```python
from build123d import *

# Parameters (mm, degrees)
BASE_FLANGE1_DEPTH             = 17.5
EDGE_FLANGE1_STRIP_W           = 4.4196
EDGE_FLANGE1_STRIP_H           = 0.7366
EDGE_FLANGE1_STRIP_CUT_DEPTH   = 445.0536
EDGE_FLANGE1_DEPTH             = 445.0536
EDGE_FLANGE2_STRIP_W           = 4.4196
EDGE_FLANGE2_STRIP_H           = 0.7366
EDGE_FLANGE2_STRIP_CUT_DEPTH   = 445.0536
EDGE_FLANGE2_DEPTH             = 445.0536
CUT_EXTRUDE1_DEPTH             = 512.790467768
CUT_EXTRUDE1_DEPTH_BACK        = 512.790467768
SKETCH16_R                     = 2
EDGE_FLANGE3_STRIP_W           = 4.4196
EDGE_FLANGE3_STRIP_H           = 0.7366
EDGE_FLANGE3_STRIP_CUT_DEPTH   = 97.7902
EDGE_FLANGE3_STRIP_2_W         = 4.4196
EDGE_FLANGE3_STRIP_2_H         = 0.7366
EDGE_FLANGE3_STRIP_CUT_2_DEPTH = 97.7902
EDGE_FLANGE3_DEPTH             = 97.7902
EDGE_FLANGE3_BEND_DEPTH        = 97.7902
EDGE_FLANGE4_STRIP_W           = 4.4196
EDGE_FLANGE4_STRIP_H           = 0.7366
EDGE_FLANGE4_STRIP_CUT_DEPTH   = 97.7902
EDGE_FLANGE4_STRIP_2_W         = 4.4196
EDGE_FLANGE4_STRIP_2_H         = 0.7366
EDGE_FLANGE4_STRIP_CUT_2_DEPTH = 97.7902
EDGE_FLANGE4_DEPTH             = 97.7902
EDGE_FLANGE4_BEND_DEPTH        = 97.7902
FILLET1_R                      = 5
FILLET2_R                      = 3
CUT_EXTRUDE2_DEPTH             = 271.508951016
CUT_EXTRUDE2_DEPTH_BACK        = 271.508951016
SKETCH29_R                     = 2.5
CUT_EXTRUDE3_DEPTH             = 271.508951016
CUT_EXTRUDE3_DEPTH_BACK        = 271.508951016
SKETCH30_R                     = 1


# Sheet-metal steps are written as plain solids
with BuildPart() as part:
    # Sketch1 → Base-Flange1 (new, symmetric)
    with BuildSketch(Plane.XY):
        with BuildLine():
            Line((-250, 74), (-250, 99.2634))
            ThreePointArc((-250, 99.2634), (-249.784254855, 99.784254855), (-249.2634, 100))
            Line((-249.2634, 100), (-224.7366, 100))
            ThreePointArc((-224.7366, 100), (-224.215745145, 99.784254855), (-224, 99.2634))
            Line((-224, 99.2634), (-224, 1.4732))
            ThreePointArc((-224, 1.4732), (-223.56850971, 0.43149029), (-222.5268, 0))
            Line((-222.5268, 0), (222.5268, 0))
            ThreePointArc((222.5268, 0), (223.56850971, 0.43149029), (224, 1.4732))
            Line((224, 1.4732), (224, 99.2634))
            ThreePointArc((224, 99.2634), (224.215745145, 99.784254855), (224.7366, 100))
            Line((224.7366, 100), (249.2634, 100))
            ThreePointArc((249.2634, 100), (249.784254855, 99.784254855), (250, 99.2634))
            Line((250, 99.2634), (250, 74))
            Line((250, 74), (250.7366, 74))
            Line((250.7366, 74), (250.7366, 99.2634))
            ThreePointArc((250.7366, 99.2634), (250.30510971, 100.30510971), (249.2634, 100.7366))
            Line((249.2634, 100.7366), (224.7366, 100.7366))
            ThreePointArc((224.7366, 100.7366), (223.69489029, 100.30510971), (223.2634, 99.2634))
            Line((223.2634, 99.2634), (223.2634, 1.4732))
            ThreePointArc((223.2634, 1.4732), (223.047654855, 0.952345145), (222.5268, 0.7366))
            Line((222.5268, 0.7366), (-222.5268, 0.7366))
            ThreePointArc((-222.5268, 0.7366), (-223.047654855, 0.952345145), (-223.2634, 1.4732))
            Line((-223.2634, 1.4732), (-223.2634, 99.2634))
            ThreePointArc((-223.2634, 99.2634), (-223.69489029, 100.30510971), (-224.7366, 100.7366))
            Line((-224.7366, 100.7366), (-249.2634, 100.7366))
            ThreePointArc((-249.2634, 100.7366), (-250.30510971, 100.30510971), (-250.7366, 99.2634))
            Line((-250.7366, 99.2634), (-250.7366, 74))
            Line((-250.7366, 74), (-250, 74))
        make_face()
    extrude(amount=BASE_FLANGE1_DEPTH, both=True)

    # Edge-Flange1 strip (across the edge) → Edge-Flange1 strip cut (cut)
    with BuildSketch(Plane(origin=(222.5268, 0, 17.5), x_dir=(0, 0, -1), z_dir=(-1, 0, 0))):
        with Locations((-0.7366, -0.3683)):
            Rectangle(EDGE_FLANGE1_STRIP_W, EDGE_FLANGE1_STRIP_H)
    extrude(amount=EDGE_FLANGE1_STRIP_CUT_DEPTH, mode=Mode.SUBTRACT)

    # Edge-Flange1 section (across the edge) → Edge-Flange1 (add)
    with BuildSketch(Plane(origin=(222.5268, 0, 17.5), x_dir=(0, 0, -1), z_dir=(-1, 0, 0))):
        with BuildLine():
            Line((0, 0.7366), (0, 9.2634))
            Line((0, 9.2634), (0.7366, 9.2634))
            Line((0.7366, 9.2634), (0.7366, 0.7366))
            ThreePointArc((0.7366, 0.7366), (0.952345145, 0.215745145), (1.4732, 0))
            Line((1.4732, 0), (1.4732, -0.7366))
            ThreePointArc((1.4732, -0.7366), (0.43149029, -0.30510971), (0, 0.7366))
        make_face()
    extrude(amount=EDGE_FLANGE1_DEPTH)

    # Edge-Flange2 strip (across the edge) → Edge-Flange2 strip cut (cut)
    with BuildSketch(Plane(origin=(-222.5268, 0, -17.5), x_dir=(0, 0, 1), z_dir=(1, 0, 0))):
        with Locations((-0.7366, -0.3683)):
            Rectangle(EDGE_FLANGE2_STRIP_W, EDGE_FLANGE2_STRIP_H)
    extrude(amount=EDGE_FLANGE2_STRIP_CUT_DEPTH, mode=Mode.SUBTRACT)

    # Edge-Flange2 section (across the edge) → Edge-Flange2 (add)
    with BuildSketch(Plane(origin=(-222.5268, 0, -17.5), x_dir=(0, 0, 1), z_dir=(1, 0, 0))):
        with BuildLine():
            Line((0, 0.7366), (0, 9.2634))
            Line((0, 9.2634), (0.7366, 9.2634))
            Line((0.7366, 9.2634), (0.7366, 0.7366))
            ThreePointArc((0.7366, 0.7366), (0.952345145, 0.215745145), (1.4732, 0))
            Line((1.4732, 0), (1.4732, -0.7366))
            ThreePointArc((1.4732, -0.7366), (0.43149029, -0.30510971), (0, 0.7366))
        make_face()
    extrude(amount=EDGE_FLANGE2_DEPTH)

    # Sketch16 → Cut-Extrude1 (cut, two sides: drawn at the far end of the back side and taken through both)
    with BuildSketch(Plane(origin=(250.7366, 0, 0), x_dir=(0, 0, -1), z_dir=(1, 0, 0)).offset(-CUT_EXTRUDE1_DEPTH_BACK)):
        with Locations(Location((0, 88.7366, 0), (0, 0, 180))):
            Circle(SKETCH16_R)
    extrude(amount=CUT_EXTRUDE1_DEPTH + CUT_EXTRUDE1_DEPTH_BACK, mode=Mode.SUBTRACT)

    # Edge-Flange3 strip (across the edge) → Edge-Flange3 strip cut (cut)
    with BuildSketch(Plane(origin=(-223.2634, 99.2634, 17.5), x_dir=(0, 0, -1), z_dir=(0, -1, 0))):
        with Locations((-0.7366, -0.3683)):
            Rectangle(EDGE_FLANGE3_STRIP_W, EDGE_FLANGE3_STRIP_H)
    extrude(amount=EDGE_FLANGE3_STRIP_CUT_DEPTH, mode=Mode.SUBTRACT)

    # Edge-Flange3 strip 2 (across the edge) → Edge-Flange3 strip cut 2 (cut)
    with BuildSketch(Plane(origin=(-223.2634, 1.4732, -17.5), x_dir=(0, 0, 1), z_dir=(0, 1, 0))):
        with Locations((-0.7366, -0.3683)):
            Rectangle(EDGE_FLANGE3_STRIP_2_W, EDGE_FLANGE3_STRIP_2_H)
    extrude(amount=EDGE_FLANGE3_STRIP_CUT_2_DEPTH, mode=Mode.SUBTRACT)

    # Edge-Flange3 section (across the edge) → Edge-Flange3 (add)
    with BuildSketch(Plane(origin=(-223.2634, 99.2634, 17.5), x_dir=(0, 0, -1), z_dir=(0, -1, 0))):
        with BuildLine():
            Line((0, 0.7366), (0, 9.2634))
            Line((0, 9.2634), (0.7366, 9.2634))
            Line((0.7366, 9.2634), (0.7366, 0.7366))
            ThreePointArc((0.7366, 0.7366), (0.952345145, 0.215745145), (1.4732, 0))
            Line((1.4732, 0), (1.4732, -0.7366))
            ThreePointArc((1.4732, -0.7366), (0.43149029, -0.30510971), (0, 0.7366))
        make_face()
    extrude(amount=EDGE_FLANGE3_DEPTH)

    # Edge-Flange3 section 2 (across the edge) → Edge-Flange3 bend (add)
    with BuildSketch(Plane(origin=(-223.2634, 1.4732, -17.5), x_dir=(0, 0, 1), z_dir=(0, 1, 0))):
        with BuildLine():
            Line((0, 0.7366), (0, 9.2634))
            Line((0, 9.2634), (0.7366, 9.2634))
            Line((0.7366, 9.2634), (0.7366, 0.7366))
            ThreePointArc((0.7366, 0.7366), (0.952345145, 0.215745145), (1.4732, 0))
            Line((1.4732, 0), (1.4732, -0.7366))
            ThreePointArc((1.4732, -0.7366), (0.43149029, -0.30510971), (0, 0.7366))
        make_face()
    extrude(amount=EDGE_FLANGE3_BEND_DEPTH)

    # Edge-Flange4 strip (across the edge) → Edge-Flange4 strip cut (cut)
    with BuildSketch(Plane(origin=(223.2634, 1.4732, 17.5), x_dir=(0, 0, -1), z_dir=(0, 1, 0))):
        with Locations((-0.7366, -0.3683)):
            Rectangle(EDGE_FLANGE4_STRIP_W, EDGE_FLANGE4_STRIP_H)
    extrude(amount=EDGE_FLANGE4_STRIP_CUT_DEPTH, mode=Mode.SUBTRACT)

    # Edge-Flange4 strip 2 (across the edge) → Edge-Flange4 strip cut 2 (cut)
    with BuildSketch(Plane(origin=(223.2634, 99.2634, -17.5), x_dir=(0, 0, 1), z_dir=(0, -1, 0))):
        with Locations((-0.7366, -0.3683)):
            Rectangle(EDGE_FLANGE4_STRIP_2_W, EDGE_FLANGE4_STRIP_2_H)
    extrude(amount=EDGE_FLANGE4_STRIP_CUT_2_DEPTH, mode=Mode.SUBTRACT)

    # Edge-Flange4 section (across the edge) → Edge-Flange4 (add)
    with BuildSketch(Plane(origin=(223.2634, 1.4732, 17.5), x_dir=(0, 0, -1), z_dir=(0, 1, 0))):
        with BuildLine():
            Line((0, 0.7366), (0, 9.2634))
            Line((0, 9.2634), (0.7366, 9.2634))
            Line((0.7366, 9.2634), (0.7366, 0.7366))
            ThreePointArc((0.7366, 0.7366), (0.952345145, 0.215745145), (1.4732, 0))
            Line((1.4732, 0), (1.4732, -0.7366))
            ThreePointArc((1.4732, -0.7366), (0.43149029, -0.30510971), (0, 0.7366))
        make_face()
    extrude(amount=EDGE_FLANGE4_DEPTH)

    # Edge-Flange4 section 2 (across the edge) → Edge-Flange4 bend (add)
    with BuildSketch(Plane(origin=(223.2634, 99.2634, -17.5), x_dir=(0, 0, 1), z_dir=(0, -1, 0))):
        with BuildLine():
            Line((0, 0.7366), (0, 9.2634))
            Line((0, 9.2634), (0.7366, 9.2634))
            Line((0.7366, 9.2634), (0.7366, 0.7366))
            ThreePointArc((0.7366, 0.7366), (0.952345145, 0.215745145), (1.4732, 0))
            Line((1.4732, 0), (1.4732, -0.7366))
            ThreePointArc((1.4732, -0.7366), (0.43149029, -0.30510971), (0, 0.7366))
        make_face()
    extrude(amount=EDGE_FLANGE4_BEND_DEPTH)

    # Fillet1
    fillet1_edges = [part.edges().sort_by_distance(p)[0] for p in [
        (222.5268, -9.2634, 17.1317),
        (-222.5268, -9.2634, 17.1317),
        (-222.5268, -9.2634, -17.1317),
        (222.5268, -9.2634, -17.1317),
        (-214, 99.2634, 17.1317),
        (250.3683, 74, -17.5),
        (-214, 99.2634, -17.1317),
        (-250.3683, 74, -17.5),
        (214, 99.2634, 17.1317),
        (214, 99.2634, -17.1317),
        (250.3683, 74, 17.5),
        (-250.3683, 74, 17.5),
    ]]
    fillet(fillet1_edges, radius=FILLET1_R)

    # Fillet2
    fillet2_edges = [part.edges().sort_by_distance(p)[0] for p in [
        (-214, 1.4732, 17.1317),
        (-214, 1.4732, -17.1317),
        (214, 1.4732, 17.1317),
        (214, 1.4732, -17.1317),
    ]]
    fillet(fillet2_edges, radius=FILLET2_R)

    # Sketch29 → Cut-Extrude2 (cut, two sides: drawn at the far end of the back side and taken through both)
    with BuildSketch(Plane(origin=(0, 0.7366, 0), x_dir=(1, 0, 0), z_dir=(0, 1, 0)).offset(-CUT_EXTRUDE2_DEPTH_BACK)):
        with Locations(Location((-26.25, 0, 0), (0, 0, 90))):
            Circle(SKETCH29_R)
        with Locations(Location((26.25, 0, 0), (0, 0, 90))):
            Circle(SKETCH29_R)
    extrude(amount=CUT_EXTRUDE2_DEPTH + CUT_EXTRUDE2_DEPTH_BACK, mode=Mode.SUBTRACT)

    # Sketch30 → Cut-Extrude3 (cut, two sides: drawn at the far end of the back side and taken through both)
    with BuildSketch(Plane(origin=(0, 0.7366, 0), x_dir=(1, 0, 0), z_dir=(0, 1, 0)).offset(-CUT_EXTRUDE3_DEPTH_BACK)):
        with Locations(Location((-14.1, 14.1, 0), (0, 0, 90))):
            Circle(SKETCH30_R)
        with Locations(Location((14.1, 14.1, 0), (0, 0, 90))):
            Circle(SKETCH30_R)
        with Locations(Location((14.1, -14.1, 0), (0, 0, 90))):
            Circle(SKETCH30_R)
        with Locations(Location((-14.1, -14.1, 0), (0, 0, 90))):
            Circle(SKETCH30_R)
    extrude(amount=CUT_EXTRUDE3_DEPTH + CUT_EXTRUDE3_DEPTH_BACK, mode=Mode.SUBTRACT)


solid = part.part
```
Work out the finished part from the listing and answer in its coordinate system (mm). A direction names the side the tool comes from. Give positions to 0.01 mm unless a question says otherwise; leave off trailing zeros. Loops run counter-clockwise (first coordinate to the right, second up) from the corner with the lowest first, then second, coordinate; pieces in that order, holes last. Notation, with made-up numbers: (46.25, 60.5) -> (100.25, 60.5) arc R21 ccw to (100.25, 89.5) -> close; hole circle Ø9 at (11, 66.25). An arc over 180 degrees is marked (long way). Put each result on its own line as item: value. Start each with the question number.
Item 1: The mould has two halves that part along Z. Classify faces 4 (the face through (-218, 51, 16.763)), 5 (the face through (218, 51, -17.5)), 6 (the face through (-224, 51, 0)): released by +Z, released by -Z, zero draft, split by the parting line, or undercut.
Item 2: Which of the six approach directions +Z, -Z, +X, -X, +Y, -Y give full straight-line access (tool end or side, diameter ignored) to faces 1 (the face through (250, 84, 0)), 2 (the face through (-3, -5, -16.763)), 3 (the face through (-218, 50, -16.763))?
Item 3: The part is cut by section C-C (x = 167). Give the vertices of the cut face in (y, z), then the cut area to 3 significant figures.
Item 4: Each of these flat-tipped pins is pushed along its axis until it touches: P1, Ø1.2, axis at y = -2, z = -16.5, coming from the -X side; P2, Ø5, axis at x = 59.5, z = 1.5, coming from the -Y side; P3, Ø0.7, axis at y = -3, z = -17, coming from the +X side; P4, Ø1.6, axis at x = -14.1, z = -14.1, coming from the -Y side. Where does it stop, or does it pass through?
Item 5: The part is cut by section A-A (y = 27.5). Give the vertices of the cut face in (x, z), then the cut area to 3 significant figures.
Item 6: Find the intervals of material crossed by L1, parallel to X at y = 81, z = 8; L2, parallel to X at y = 0.2, z = 0; L3, parallel to X at y = 63.5, z = 12.5, in increasing order. Write a range as [from, to].
Item 7: The part is cut by section B-B (z = 7). Give the vertices of the cut face in (x, y).
Answers below:
1. face 4: undercut
1. face 5: released by -Z
1. face 6: zero draft
2. face 1: +Z, -Z, -Y
2. face 2: +X, -X, -Y
2. face 3: +Y
3. outline: (-9.26, -17.5) -> (-0.74, -17.5) arc R1.47 ccw to (0.74, -16.03) -> (0.74, 16.03) arc R1.47 ccw to (-0.74, 17.5) -> (-9.26, 17.5) -> (-9.26, 16.76) -> (-0.74, 16.76) arc R0.74 cw to (0, 16.03) -> (0, -16.03) arc R0.74 cw to (-0.74, -16.76) -> (-9.26, -16.76) -> close
3. area: 38.7 mm2
4. P1: x = -222.53
4. P2: y = 0
4. P3: x = 222.53
4. P4: through
5. outline: (-224, -16.03) arc R1.47 ccw to (-222.53, -17.5) -> (-214, -17.5) -> (-214, -16.76) -> (-222.53, -16.76) arc R0.74 cw to (-223.26, -16.03) -> (-223.26, 16.03) arc R0.74 cw to (-222.53, 16.76) -> (-214, 16.76) -> (-214, 17.5) -> (-222.53, 17.5) arc R1.47 ccw to (-224, 16.03) -> close; (214, -17.5) -> (222.53, -17.5) arc R1.47 ccw to (224, -16.03) -> (224, 16.03) arc R1.47 ccw to (222.53, 17.5) -> (214, 17.5) -> (214, 16.76) -> (222.53, 16.76) arc R0.74 cw to (223.26, 16.03) -> (223.26, -16.03) arc R0.74 cw to (222.53, -16.76) -> (214, -16.76) -> close
5. area: 77.5 mm2
6. L1: [-250.74, -250], [-224, -223.26], [223.26, 224], [250, 250.74]
6. L2: [-223.27, -28.75], [-23.75, 23.75], [28.75, 223.27]
6. L3: [-224, -223.26], [223.26, 224]
7. outline: (-250.74, 74) -> (-250, 74) -> (-250, 99.26) arc R0.74 cw to (-249.26, 100) -> (-224.74, 100) arc R0.74 cw to (-224, 99.26) -> (-224, 1.47) arc R1.47 ccw to (-222.53, 0) -> (222.53, 0) arc R1.47 ccw to (224, 1.47) -> (224, 99.26) arc R0.74 cw to (224.74, 100) -> (249.26, 100) arc R0.74 cw to (250, 99.26) -> (250, 74) -> (250.74, 74) -> (250.74, 99.26) arc R1.47 ccw to (249.26, 100.74) -> (224.74, 100.74) arc R1.47 ccw to (223.26, 99.26) -> (223.26, 1.47) arc R0.74 cw to (222.53, 0.74) -> (-222.53, 0.74) arc R0.74 cw to (-223.26, 1.47) -> (-223.26, 99.26) arc R1.47 ccw to (-224.74, 100.74) -> (-249.26, 100.74) arc R1.47 ccw to (-250.74, 99.26) -> close
